from build123d import *

# Parameters (mm, degrees)
F0_R     = 0.75
F1_DEPTH = 25
F5_R     = 0.75
F7_R     = 0.3


with BuildPart() as f1:
    # F0 (on Top) → F1 (new body)
    with BuildSketch(Plane.XY):
        Circle(F0_R)
    extrude(amount=F1_DEPTH)

    # F6: sweep along a path in F4
    with BuildLine(Plane.YZ) as f6_path:
        add(Plane.YZ * Edge.make_bspline(
            [(0, 25), (0.0276527047, 25.5188264102), (0.048108405, 26.7957580563), (1.2597410469, 28.3543405458), (1.3940753419, 28.5497736832), (1.4285740908, 28.5981334746)],
            knots=[0, 0, 0, 0, 0.4186868784, 0.8442205829, 1, 1, 1, 1], degree=3))
    # F5 (on offset) → F6 (sweep)
    with BuildSketch(Plane.XY.offset(25)):
        Circle(F5_R)
    sweep(path=f6_path.line)

    # F7
    f7_edges = [f1.edges().sort_by_distance(p)[0] for p in [
        (-0.75, 1.428574, 28.598133),
    ]]
    fillet(f7_edges, radius=F7_R)


solid = f1.part
Can you work these out from the model? Positions are in its coordinate system, mm. A direction names the side the tool comes from. Give positions to 0.01 mm unless a question says otherwise; leave off trailing zeros. Order: outer loops, then holes, each group sorted by start corner. A loop starts at its lowest first (then second) coordinate and runs counter-clockwise, first axis right, second up. Notation, with made-up numbers: M 23.25,-12 L 76.25,-12 A21 ccw 76.25,21 Z; hole C -19.5,61 d4. An arc over 180 degrees is marked long. Use a Markdown table: item, result. Add a question column.
Item 1: For faces 1 (the flat face through (0, 0, 0)), 2 (the cylindrical face through (-0.75, 0.03, 12.32)), which set-ups out of +Z, -Z, +X, -X, +Y, -Y let a thin tool reach every point of the face, with its end or its side?
Item 2: Suppose I cut it at A-A (z = 9.75). List the corners of the cut face in (x, y) for me, then the cut area to 3 significant figures.
Item 3: If I drill on L1, parallel to Y at x = 0.1, z = 2.5; L2, parallel to Y at x = -0.6, z = 15.75; L3, parallel to Z at x = -0.4, y = -0.1, over which ranges is the centre line in solid material (lowest first)? Write a range as [from, to].
Item 4: Will this pin go through, and if not, where does the flat tip stop? pin 1 (1.5 mm diameter, centred on y = 1, z = 7, fed in from -X).
Answer sheet:
| question | item | result |
|---|---|---|
| 1 | face 1 | -Z, +X, -X, +Y, -Y |
| 1 | face 2 | -Z |
| 2 | outline | C 0,0 d1.5 |
| 2 | area | 1.77 mm² |
| 3 | L1 | y = [-0.74, 0.74] |
| 3 | L2 | y = [-0.45, 0.45] |
| 3 | L3 | z = [0, 27.45] |
| 4 | pin 1 | stops at x = -0.71 |
